```python
from build123d import *

# Parameters (mm, degrees)
SKETCH6_W           = 40
SKETCH6_H           = 20
BOSS_EXTRUDE3_DEPTH = 19.854784811
SKETCH9_W           = 10
SKETCH9_H           = 20
CUT_EXTRUDE6_DEPTH  = 15
SKETCH10_R          = 4
CUT_EXTRUDE7_DEPTH  = 15
SKETCH11_R          = 2
CUT_EXTRUDE8_DEPTH  = 5
FILLET1_R           = 10
FILLET2_R           = 10
FILLET5_R           = 3


with BuildPart() as part:
    # Sketch6 → Boss-Extrude3 (new body)
    with BuildSketch(Plane.XY):
        Rectangle(SKETCH6_W, SKETCH6_H)
    extrude(amount=BOSS_EXTRUDE3_DEPTH)

    # Sketch9 → Cut-Extrude6 (cut)
    with BuildSketch(Plane.XY.offset(19.854784811)):
        with Locations((-15, 0)):
            Rectangle(SKETCH9_W, SKETCH9_H)
        with Locations((15, 0)):
            Rectangle(SKETCH9_W, SKETCH9_H)
    extrude(amount=-CUT_EXTRUDE6_DEPTH, mode=Mode.SUBTRACT)

    # Sketch10 → Cut-Extrude7 (cut)
    with BuildSketch(Plane.XZ.offset(10)):
        with Locations(Location((0, 12.5, 0), (0, 0, 270))):
            Circle(SKETCH10_R)
    extrude(amount=-CUT_EXTRUDE7_DEPTH, mode=Mode.SUBTRACT)

    # Sketch11 → Cut-Extrude8 (cut)
    with BuildSketch(Plane.XY.offset(4.854784811)):
        with Locations((-15, 0)):
            Circle(SKETCH11_R)
        with Locations((15, 0)):
            Circle(SKETCH11_R)
    extrude(amount=-CUT_EXTRUDE8_DEPTH, mode=Mode.SUBTRACT)

    # Fillet1
    fillet1_edges = [part.edges().sort_by_distance(p)[0] for p in [
        (10, 0, 19.854784811),
    ]]
    fillet(fillet1_edges, radius=FILLET1_R)

    # Fillet2
    fillet2_edges = [part.edges().sort_by_distance(p)[0] for p in [
        (-10, 0, 19.854784811),
    ]]
    fillet(fillet2_edges, radius=FILLET2_R - 0.0001)  # a hair under: the kernel refuses the full size

    # Fillet5
    fillet5_edges = [part.edges().sort_by_distance(p)[0] for p in [
        (-10, 0, 4.854784811),
        (10, 0, 4.854784811),
    ]]
    fillet(fillet5_edges, radius=FILLET5_R - 0.0001)  # a hair under: the kernel refuses the full size


solid = part.part
```
Model file for the job. Use its own axes, mm. A direction names the side the tool comes from. Coordinates: 2 decimals unless noted, no trailing zeros. Write each loop counter-clockwise with the first axis right and the second up, starting at its lowest first coordinate (ties: lowest second). Pieces come first, ordered by that corner, then holes. Notation, with made-up numbers: (61, -36.5) - (89, -36.5) arc R25 cw to (89, 1.5) - close; hole circle Ø3 at (-16, -34.75). An arc over 180 degrees is marked (long way). One line per item, written item: value. Start each with the question number.
1. Slice it at A-A (y = 0). Count the separate pieces of the cut face and the enclosed holes in it, plus the area to 3 significant figures.
2. Flat gauge pins, fed straight in: pin 1 (1.5 mm diameter, centred on y = -4.5, z = 13, fed in from +X); pin 2 (1 mm diameter, centred on y = 2.5, z = 13.5, fed in from +X); pin 3 (0.6 mm diameter, centred on y = 0.5, z = 8.5, fed in from -X). Where does each tip first touch, or does it go through?
3. Probe line 1 (Y direction, x = 15, z = 3.35); line 2 (Z direction, x = 3, y = 4); line 3 (Z direction, x = 14.5, y = 3.75). List the from-to ranges inside material, lowest first. Write a range as from..to.
4. Tool access for faces 5 (the flat face through (-10, 0, 9)), 6 (the flat face through (17.2, 0.1, 4.855)), 7 (the cylindrical face through (-2.4, -2.6, 15.7)): list every direction of +Z, -Z, +X, -X, +Y, -Y with a clear straight run to the whole face (end or side of a thin tool).
5. Slice it at B-B (x = 15). Write the cut outline in (y, z), plus the area to 3 significant figures.
6. Mould opens along Z. For faces 1 (the flat face through (-17.3, 0.1, 4.855)), 2 (the cylindrical face through (13.4, -1.2, 2.5)), 3 (the flat face through (0, 5, 13)), 4 (the flat face through (0, 0, 0)) say: released by +Z, released by -Z, zero draft, split by the parting line, or undercut.
Answers below:
1. separate pieces: 3
1. enclosed holes: 1
1. area: 366 mm^2
2. pin 1: stops at x = 9.71
2. pin 2: stops at x = 9.49
2. pin 3: stops at x = -10
3. line 1: y = -10..-2, 2..10
3. line 2: z = 0..9.85, 15.15..19.39
3. line 3: z = 0..4.85
4. face 5: +Z, -X, +Y, -Y
4. face 6: +Z, +X, +Y, -Y
4. face 7: -Y
5. outline: (-10, 0) - (-2, 0) - (-2, 4.85) - (-10, 4.85) - close; (2, 0) - (10, 0) - (10, 4.85) - (2, 4.85) - close
5. area: 77.7 mm^2
6. face 1: released by +Z
6. face 2: zero draft
6. face 3: undercut
6. face 4: released by -Z
